```python
from build123d import *

# Parameters (mm, degrees)
F1_DEPTH = 12.7
F2_SIZE  = 12.69999
F4_D     = 6.35


# Not quite as in the source:
# - a fillet or chamfer is up to 0.001 mm smaller than in the source, because OpenCascade refuses the exact size


with BuildPart() as f1:
    # F0 (on Top) → F1 (new body)
    with BuildSketch(Plane.XY):
        Polygon((9.0852697523, 24.0329056978), (-11.2347302477, 24.0329056978), (-11.2347302477, 0), (-11.2347302477, -37.6667892456), (0, -52.1670943022), (9.0852697523, -33.5160031522), align=None)
    extrude(amount=F1_DEPTH)

    # F2 (size 12.7 in the source; OpenCascade refuses exactly that, so slightly less here)
    f2_edges = [f1.edges().sort_by_distance(p)[0] for p in [
        (-11.23473, -6.816942, 12.7),
    ]]
    chamfer(f2_edges, length=F2_SIZE)

    # F4 (through all)
    with Locations(Plane.XY.offset(12.7)):
        with Locations((3.3710829448, 14.6072776988)):
            Hole(F4_D / 2)


solid = f1.part
```
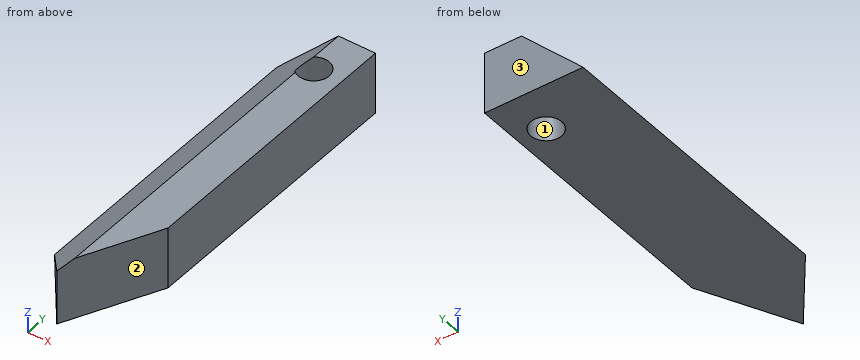
Check sheet for the modelled part. Datum: model origin and axes. Units: mm. Face numbers are marked on the shaded views. Coordinates: 2 decimals unless noted, no trailing zeros. Write each loop counter-clockwise with the first axis right and the second up, starting at its lowest first coordinate (ties: lowest second). Pieces come first, ordered by that corner, then holes. Notation, with made-up numbers: M 89.25,69 L 106.25,69 A23 cw 106.25,92 Z; hole C 86.5,78.5 d2. An arc over 180 degrees is marked long. Write item = value, one per line. Start each with the question number.
1. Mould release check, pull along X, two halves, no side actions. Record for the marked faces 1, 2 and 3: pulls with the +X half, pulls with the -X half, needs draft (parallel to the pull), parting line crosses it, or undercut.
2. Thickness scan on probe 1 along X at (y, z) = (19.5, 11.25); probe 2 along Y at (x, z) = (2, 2); probe 3 along Y at (x, z) = (4.25, 3). Record the ranges inside material, lowest first.
3. Sectioned sample at B-B (z = 8.25). Record the cut outline in (x, y) (3 decimals).
4. Go/stop test with flat-tipped pins: pin 1 (3 mm diameter, centred on x = -7.5, z = 3, fed in from -Y); pin 2 (1.5 mm diameter, centred on x = -5, z = 5, fed in from -Y); pin 3 (3 mm diameter, centred on x = 6, z = 4.5, fed in from -Y). Record where each tip stops, or that it passes through.
5. Sectioned sample at D-D (x = -5). Record the cut outline in (y, z), then the cut area to 3 significant figures.
6. Sectioned sample at A-A (x = 3). Record the cut outline in (y, z), then the cut area to 3 significant figures.
The answers:
q1.face_1 = undercut
q1.face_2 = pulls with the +X half
q1.face_3 = needs draft
q2.probe_1 = 0.02 to 9.09
q2.probe_2 = -48.06 to 11.74, 17.47 to 24.03
q2.probe_3 = -43.44 to 11.56, 17.66 to 24.03
q3.outline = M -2.985,-48.315 L 0,-52.167 L 9.085,-33.516 L 9.085,24.033 L -2.985,24.033 Z; hole C 3.371,14.607 d6.35
q4.pin_1 = -44.42
q4.pin_2 = -46.68
q4.pin_3 = -42.93
q5.outline = M -45.71,0 L 24.03,0 L 24.03,6.23 L -45.71,6.23 Z
q5.area = 435 mm²
q6.outline = M -46.01,0 L 11.45,0 L 11.45,12.7 L -46.01,12.7 Z; M 17.76,0 L 24.03,0 L 24.03,12.7 L 17.76,12.7 Z
q6.area = 809 mm²
